Part print with two shaded views. Sizes in mm from the minimum x, y, z corner. A direction names the side the tool comes from. Round coordinates to 2 decimals unless told otherwise and drop trailing zeros. Loops run counter-clockwise (first coordinate to the right, second up) from the corner with the lowest first, then second, coordinate; pieces in that order, holes last.
(1) Flat gauge pins, fed straight in: pin 1 (10 mm diameter, centred on x = 29, z = 14.5, fed in from +Y); pin 2 (3 mm diameter, centred on x = 37, y = 6, fed in from +Z); pin 3 (3 mm diameter, centred on x = 25.5, y = 15.5, fed in from -Z); pin 4 (3 mm diameter, centred on x = 41.75, z = 30.75, fed in from -Y). Where does each tip first touch, or does it go through?
(2) Cut at B-B on x = 3.25. List the corners of the cut face in (y, z).
(3) Tool access for the marked faces 1, 2, 3, 4 and 5: list every direction of +Z, -Z, +X, -X, +Y, -Y with a clear straight run to the whole face (end or side of a thin tool).
(4) Cut at A-A on z = 3.25. List the corners of the cut face in (x, y).
(5) Cut at D-D on y = 8. List the corners of the cut face in (x, z).
(6) Cut at C-C on x = 19. List the corners of the cut face in (y, z), then the cut area to 3 significant figures.
(7) Probe probe 1 along Z at (x, y) = (41.75, 0.8); probe 2 along X at (y, z) = (0.5, 3.25); probe 3 along Y at (x, z) = (36.5, 20.5). List the from-to ranges inside material, lowest first.
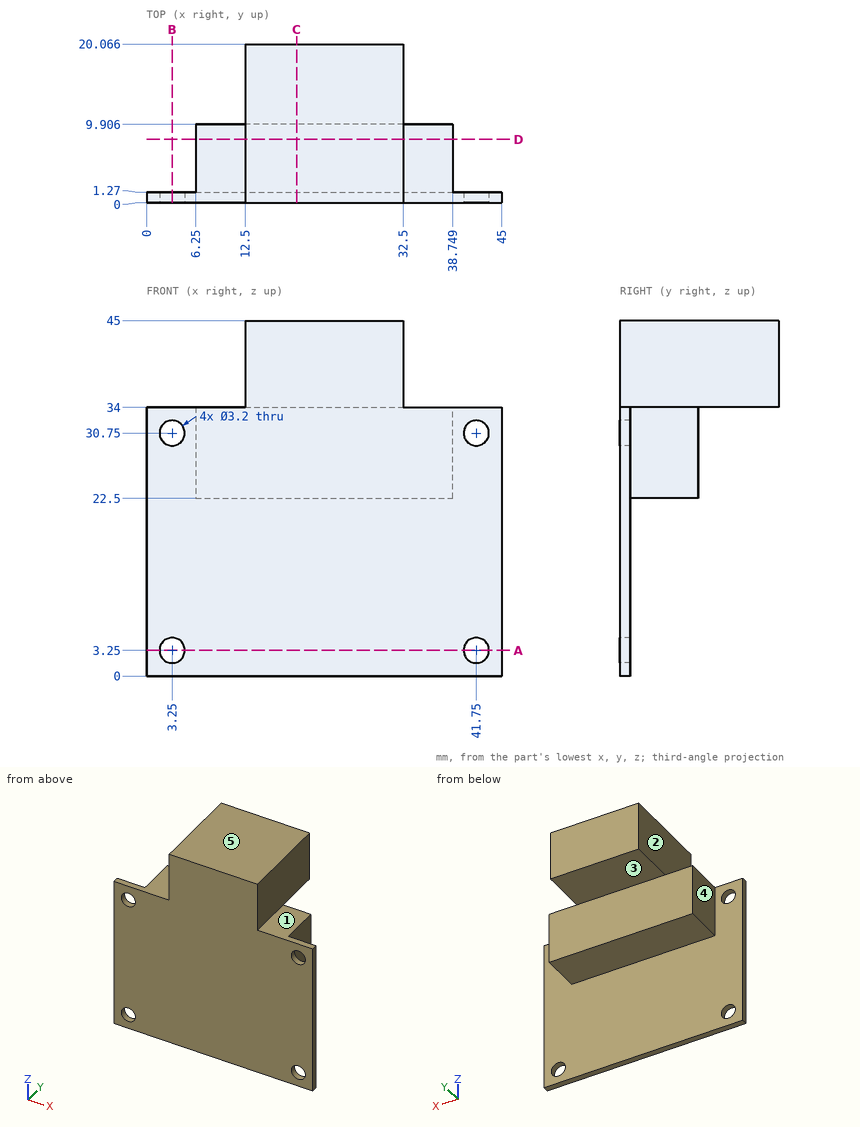
Final values:
1. pin 1: stops at y = 1.27
1. pin 2: stops at z = 34
1. pin 3: stops at z = 34
1. pin 4: passes through
2. outline: (0, 0) - (1.27, 0) - (1.27, 1.65) - (0, 1.65) - close; (0, 4.85) - (1.27, 4.85) - (1.27, 29.15) - (0, 29.15) - close; (0, 32.35) - (1.27, 32.35) - (1.27, 34) - (0, 34) - close
3. face 1: +Z, +X, +Y, -Y
3. face 2: +Z, -X, +Y, -Y
3. face 3: -Z, +X, -X, +Y
3. face 4: +Z, -Z, -X, +Y
3. face 5: +Z, +X, -X, +Y, -Y
4. outline: (0, 0) - (1.65, 0) - (1.65, 1.27) - (0, 1.27) - close; (4.85, 0) - (40.15, 0) - (40.15, 1.27) - (4.85, 1.27) - close; (43.35, 0) - (45, 0) - (45, 1.27) - (43.35, 1.27) - close
5. outline: (6.25, 22.5) - (38.75, 22.5) - (38.75, 34) - (32.5, 34) - (32.5, 45) - (12.5, 45) - (12.5, 34) - (6.25, 34) - close
6. outline: (0, 0) - (1.27, 0) - (1.27, 22.5) - (9.91, 22.5) - (9.91, 34) - (20.07, 34) - (20.07, 45) - (0, 45) - close
6. area: 363 mm2
7. probe 1: z = 0 to 1.65, 4.85 to 29.15, 32.35 to 34
7. probe 2: x = 0 to 1.65, 4.85 to 40.15, 43.35 to 45
7. probe 3: y = 0 to 1.27
